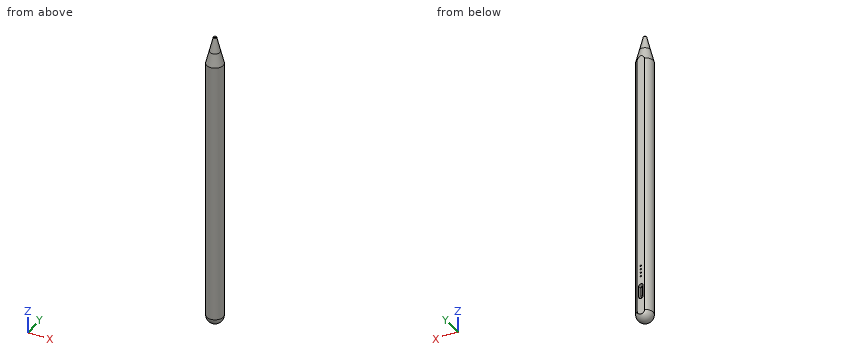
```python
from build123d import *

# Parameters (mm, degrees)
SKETCH_R        = 4.5
PAD_DEPTH       = 145.5
SKETCH001_W     = 4
SKETCH001_H     = 3.989153
POCKET_DEPTH    = 150
SKETCH002_R     = 0.4
POCKET001_DEPTH = 10
FILLET_R        = 0.2
SKETCH003_W     = 0.8
SKETCH003_H     = 7
PAD001_DEPTH    = 3
FILLET001_R     = 1


with BuildPart() as part:
    # Sketch → Pad (new body)
    with BuildSketch(Plane.XY):
        Circle(SKETCH_R)
    extrude(amount=PAD_DEPTH)

    # Cone → Cone (revolve)
    with BuildSketch(Plane(origin=(0, 0, 145.5), x_dir=(0, 1, 0), z_dir=(1, 0, 0))):
        Polygon((0, 0), (4.5, 0), (2.75, 7), (0, 7), align=None)
    revolve(axis=Axis((0, 0, 145.5), (0, 0, 1)))

    # Sphere001 → Sphere001 (revolve)
    with BuildSketch(Plane.XZ):
        with BuildLine():
            ThreePointArc((0, -4.5), (4.5, 0), (0, 4.5))
            Line((0, 4.5), (0, -4.5))
        make_face()
    revolve(axis=Axis((0, 0, 0), (0, 0, 1)))

    # Sketch001 → Pocket (cut, symmetric)
    with BuildSketch(Plane.XY):
        with Locations((0, 6.025705)):
            Rectangle(SKETCH001_W, SKETCH001_H)
    extrude(amount=POCKET_DEPTH, both=True, mode=Mode.SUBTRACT)

    # Sketch002 → Pocket001 (cut)
    with BuildSketch(Plane.XZ):
        with Locations((0, 19.9)):
            Circle(SKETCH002_R)
        with Locations((0, 21.9)):
            Circle(SKETCH002_R)
        with Locations((0, 23.9)):
            Circle(SKETCH002_R)
        with Locations((0, 25.9)):
            Circle(SKETCH002_R)
        with BuildLine():
            Line((-1.25, 14.25), (-1.25, 8.25))
            ThreePointArc((-1.25, 8.25), (0, 7), (1.25, 8.25))
            Line((1.25, 8.25), (1.25, 14.25))
            ThreePointArc((1.25, 14.25), (0, 15.5), (-1.25, 14.25))
        make_face()
    extrude(amount=-POCKET001_DEPTH, mode=Mode.SUBTRACT)

    # Cone001 → Cone001 (revolve)
    with BuildSketch(Plane(origin=(0, 0, 152.5), x_dir=(1, 0, 0), z_dir=(0, -1, 0))):
        Polygon((0, 0), (2.75, 0), (0.8, 8), (0, 8), align=None)
    revolve(axis=Axis((0, 0, 152.5), (0, 0, 1)))

    # Sphere → Sphere (revolve)
    with BuildSketch(Plane(origin=(0, 0, 160.5), x_dir=(1, 0, 0), z_dir=(0, -1, 0))):
        with BuildLine():
            ThreePointArc((0, -0.5), (0.5, 0), (0, 0.5))
            Line((0, 0.5), (0, -0.5))
        make_face()
    revolve(axis=Axis((0, 0, 160.5), (0, 0, 1)))

    # Fillet
    fillet_edges = [part.edges().sort_by_distance(p)[0] for p in [
        (-0.8, 0, 160.5),
    ]]
    fillet(fillet_edges, radius=FILLET_R)

    # Sketch003 → Pad001 (join)
    with BuildSketch(Plane.XZ):
        with Locations((0, 11.5)):
            Rectangle(SKETCH003_W, SKETCH003_H)
    extrude(amount=-PAD001_DEPTH)

    # Fillet001
    fillet001_edges = [part.edges().sort_by_distance(p)[0] for p in [
        (0, 3, 8),
        (0, 3, 15),
    ]]
    fillet(fillet001_edges, radius=FILLET001_R)


solid = part.part
```
Work out the finished part from the listing and answer in its coordinate system (mm). Round coordinates to 2 decimals unless told otherwise and drop trailing zeros. Order: outer loops, then holes, each group sorted by start corner. A loop starts at its lowest first (then second) coordinate and runs counter-clockwise, first axis right, second up.
Q1. A cutting plane is placed at A-A, the plane z = 40. Determine the outline of the cut face in (x, y), then the cut area to 3 significant figures.
Solution:
outline: (-2, 4.03) arc R4.5 ccw (long way) to (2, 4.03) - close
area: 62.4 mm2
Q2. Find the intervals of material crossed by line 1 along X through (y, z) = (1, 19.9); line 2 along X through (y, z) = (-0.5, 8); line 3 along Y through (x, z) = (0.75, 27.5), in increasing order.
Solution:
line 1: x = -4.39 to -0.4, 0.4 to 4.39
line 2: x = -4.47 to 4.47
line 3: y = -4.44 to 4.03
Q3. Given pin 1 Ø3 at (y, z) = (2.5, 12.5) entering from +X; pin 2 Ø0.6 at (x, y) = (0, 1) entering from +Z; pin 3 Ø4 at (x, z) = (-2.5, 92.5) entering from -Y; pin 4 Ø3 at (y, z) = (1.5, 12.5) entering from -X, each flat-ended and moving along its own axis, determine where each tip first touches the part or whether it passes through.
Solution:
pin 1: stops at x = 4.39
pin 2: stops at z = 160.49
pin 3: stops at y = -4.47
pin 4: stops at x = -4.5
